The model under review builds one solid part; all positions refer to its coordinate system, in mm. A direction names the side the tool comes from. Give positions to 0.01 mm unless a question says otherwise; leave off trailing zeros. Loops run counter-clockwise (first coordinate to the right, second up) from the corner with the lowest first, then second, coordinate; pieces in that order, holes last. Notation, with made-up numbers: (-30.5, 58) - (22.5, 58) arc R16 ccw to (22.5, 62) - close; hole circle Ø5 at (8, -31). An arc over 180 degrees is marked (long way). Answer as a JSON object with one key per item and string values.
from build123d import *

# Parameters (mm, degrees)
SKETCH_R        = 11.5
SKETCH_R_2      = 3.93
PAD_DEPTH       = 25.4
SKETCH001_R     = 4.9
POCKET_DEPTH    = 12.7
SKETCH002_R     = 1.7
POCKET001_DEPTH = 11.501
SKETCH003_R     = 1.7
POCKET002_DEPTH = 11.501


with BuildPart() as part:
    # Sketch → Pad (new body)
    with BuildSketch(Plane.XY):
        Circle(SKETCH_R)
        Circle(SKETCH_R_2, mode=Mode.SUBTRACT)
    extrude(amount=PAD_DEPTH)

    # Sketch001 (on Face4 of Pad) → Pocket (cut)
    with BuildSketch(Plane.XY.offset(25.4)):
        Circle(SKETCH001_R)
    extrude(amount=-POCKET_DEPTH, mode=Mode.SUBTRACT)

    # Sketch002 → Pocket001 (cut, through all)
    with BuildSketch(Plane.XZ):
        with Locations((0, 4)):
            Circle(SKETCH002_R)
        with Locations((0, 21.4)):
            Circle(SKETCH002_R)
    extrude(amount=-POCKET001_DEPTH, mode=Mode.SUBTRACT)

    # Sketch003 → Pocket002 (cut, through all)
    with BuildSketch(Plane.YZ):
        with Locations((0, 4)):
            Circle(SKETCH003_R)
        with Locations((0, 21.4)):
            Circle(SKETCH003_R)
    extrude(amount=-POCKET002_DEPTH, mode=Mode.SUBTRACT)


with BuildPart() as part_1:
    # Clone placement: moved
    add(part.part.moved(Location((0, 0, -26.4))))


solid = part_1.part
Q1. Consider section D-D, the plane y = 2.5. State the section outline as (x, z) points.
Results:
{"outline": "(-11.22, -26.4) - (-3.03, -26.4) - (-3.03, -13.7) - (-4.21, -13.7) - (-4.21, -1) - (-11.22, -1) - close; (3.03, -26.4) - (11.22, -26.4) - (11.22, -1) - (4.21, -1) - (4.21, -13.7) - (3.03, -13.7) - close"}
Q2. Consider section A-A, the plane y = 0. State the section outline as (x, z) points.
Results:
{"outline": "(-11.5, -26.4) - (-3.93, -26.4) - (-3.93, -24.1) - (-11.5, -24.1) - close; (-11.5, -20.7) - (-3.93, -20.7) - (-3.93, -13.7) - (-4.9, -13.7) - (-4.9, -6.7) - (-11.5, -6.7) - close; (-11.5, -3.3) - (-4.9, -3.3) - (-4.9, -1) - (-11.5, -1) - close; (3.93, -26.4) - (11.5, -26.4) - (11.5, -1) - (4.9, -1) - (4.9, -13.7) - (3.93, -13.7) - close"}
Q3. The part is to be moulded in two halves that separate along Z. For faces 5 (the face through (5, 0, -26.4)), 6 (the face through (-7.47, -0.37, -24.06)), 7 (the face through (5, -2, -1)), say which applies: +Z half, -Z half, draft (parallel to the pull), parting line (faces both ways), or undercut.
Results:
{"face 5": "-Z half", "face 6": "undercut", "face 7": "+Z half"}
Q4. For faces 1 (the face through (2.261, -4.347, -7.261)), 2 (the face through (-0.37, 7.47, -24.06)), 3 (the face through (1.81, -3.49, -20.14)), 4 (the face through (-8, -0.37, -6.66)), list the 3-axis set-ups (+Z, -Z, +X, -X, +Y, -Y) from which the entire face can be reached by the end or side of a thin tool; tool diameter is ignored.
Results:
{"face 1": "+Z", "face 2": "+Y", "face 3": "+Z, -Z", "face 4": "-X"}
Q5. Consider section B-B, the plane x = 0. State the section outline as (y, z) points, plus the area to 3 significant figures.
Results:
{"outline": "(-11.5, -26.4) - (-3.93, -26.4) - (-3.93, -13.7) - (-4.9, -13.7) - (-4.9, -1) - (-11.5, -1) - close; (3.93, -26.4) - (11.5, -26.4) - (11.5, -24.1) - (3.93, -24.1) - close; (3.93, -20.7) - (11.5, -20.7) - (11.5, -6.7) - (4.9, -6.7) - (4.9, -13.7) - (3.93, -13.7) - close; (4.9, -3.3) - (11.5, -3.3) - (11.5, -1) - (4.9, -1) - close", "area": "312 mm^2"}
Q6. Consider section C-C, the plane z = -4.5. State the section outline as (x, y) points, plus the area to 3 significant figures.
Results:
{"outline": "(-11.38, -1.62) arc R11.5 ccw (long way) to (1.62, 11.38) - (1.62, 4.62) arc R4.9 cw (long way) to (-4.62, -1.62) - close; (-11.38, 1.62) - (-4.62, 1.62) arc R4.9 cw to (-1.62, 4.62) - (-1.62, 11.38) arc R11.5 ccw to start", "area": "297 mm^2"}
Q7. Clearance check with flat-ended pins moving along their axes: pin 1 Ø2 at (x, z) = (-1.5, -5.5) entering from +Y; pin 2 Ø2 at (x, y) = (2, 1) entering from +Z; pin 3 Ø1 at (y, z) = (9, -23.5) entering from +X; pin 4 Ø2 at (y, z) = (0, -22.4) entering from -X. State where each tip first meets the part, or that it passes through.
Results:
{"pin 1": "stops at y = 11.46", "pin 2": "passes through", "pin 3": "stops at x = 7.75", "pin 4": "stops at x = 3.8"}
Q8. To check wall thickness, follow probe 1 along X at (y, z) = (0, -7.75); probe 2 along X at (y, z) = (0, -17). State the ranges of each line that lie inside material, in increasing order. Write a range as [from, to].
Results:
{"probe 1": "x = [-11.5, -4.9], [4.9, 11.5]", "probe 2": "x = [-11.5, -3.93], [3.93, 11.5]"}
